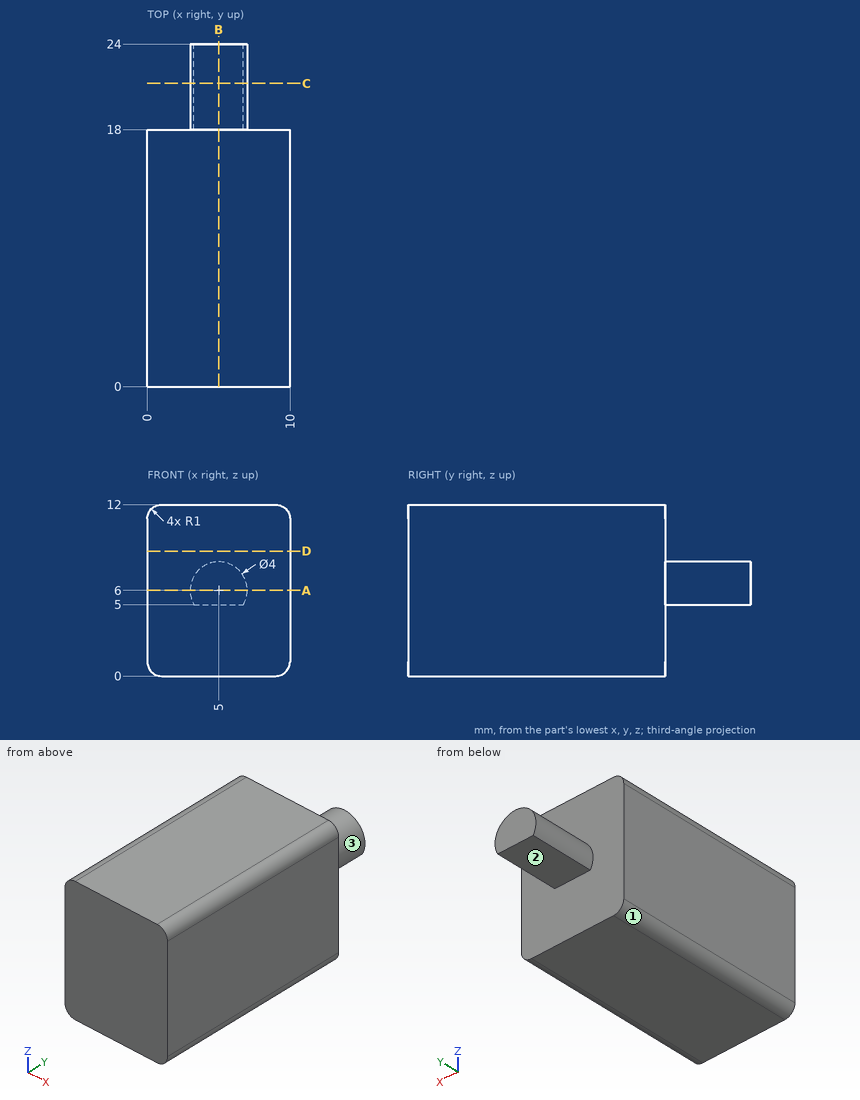
Print and shaded views of the part. All mm, measured from the part's lowest x, y and z. A direction names the side the tool comes from. Coordinates: 2 decimals unless noted, no trailing zeros. Write each loop counter-clockwise with the first axis right and the second up, starting at its lowest first coordinate (ties: lowest second). Pieces come first, ordered by that corner, then holes. Notation, with made-up numbers: (10, 79.5) - (57, 79.5) arc R32 ccw to (57, 111.5) - close; hole circle Ø2 at (-37.75, 8). An arc over 180 degrees is marked (long way). One line per question, with ' | ' between items. Start each with the question number.
Q1. Cut at B-B, the plane x = 5. List the corners of the cut face in (y, z).
Q2. 3-axis set-ups, long thin cutter, end or side, ignore diameter. For the marked faces 1, 2 and 3: which of +Z, -Z, +X, -X, +Y, -Y reach the whole face in a straight line?
Q3. Drill centre lines: line 1 (Y direction, x = 3, z = 8.5); line 2 (X direction, y = 17.5, z = 0.5); line 3 (X direction, y = 14.75, z = 11.25). Where is each one in solid material? Low to high. Write a range as [from, to].
Q4. Cut at C-C, the plane y = 21.25. List the corners of the cut face in (x, z), then the cut area to 3 significant figures.
Q5. Cut at D-D, the plane z = 8.75. List the corners of the cut face in (x, y), then the cut area to 3 significant figures.
Q6. Pin check, flat tips, straight feed: pin 1 (6 mm diameter, centred on x = 6.5, y = 5, fed in from -Z); pin 2 (3 mm diameter, centred on x = 4.5, y = 22, fed in from -Z). Stop position of each tip, or through.
Q7. Cut at A-A, the plane z = 6. List the corners of the cut face in (x, y), then the cut area to 3 significant figures.
Answer below:
1) outline: (0, 0) - (18, 0) - (18, 5) - (24, 5) - (24, 8) - (18, 8) - (18, 12) - (0, 12) - close
2) face 1: -Z, -X, +Y, -Y | face 2: -Z, +X, -X, +Y | face 3: +Y
3) line 1: [0, 18] | line 2: [0.13, 9.87] | line 3: [0.03, 9.97]
4) outline: (3.27, 5) - (6.73, 5) arc R2 ccw (long way) to start | area: 10.1 mm^2
5) outline: (0, 0) - (10, 0) - (10, 18) - (0, 18) - close | area: 180 mm^2
6) pin 1: z = 0 | pin 2: z = 5
7) outline: (0, 0) - (10, 0) - (10, 18) - (7, 18) - (7, 24) - (3, 24) - (3, 18) - (0, 18) - close | area: 204 mm^2
